Job drawing, mm, ordinate dimensions from the low corner. One solid piece. Round coordinates to 2 decimals unless told otherwise and drop trailing zeros. Write each loop counter-clockwise with the first axis right and the second up, starting at its lowest first coordinate (ties: lowest second). Pieces come first, ordered by that corner, then holes. Notation, with made-up numbers: (21, 63) -> (26, 63) arc R11 cw to (26, 83) -> close; hole circle Ø11 at (29, 5.5). An arc over 180 degrees is marked (long way). Use CSV: the item, a comma, the result in double quotes. Start each with the question number.
(1) Drop flat-ended pins along their axis: pin 1 (1.5 mm diameter, centred on y = 14.5, z = 10, fed in from +X); pin 2 (4 mm diameter, centred on x = 6.5, z = 11.5, fed in from +Y). Give the stop position or say it passes through.
(2) Saw through at A-A (z = 8.5). Give the cut face in (x, y).
(3) Saw through at C-C (y = 16.5). Give the cut face in (x, z), plus the area to 3 significant figures.
(4) Two-plate mould, pull along Z, no slides. Class the marked faces 1, 2 and 3: released by +Z, released by -Z, zero draft, split by the parting line, or undercut.
(5) Probe line 1 (Z direction, x = 2.25, y = 16.5); line 2 (Y direction, x = 0.6, z = 8.5). List the from-to ranges inside material, lowest first. Write a range as [from, to].
(6) Saw through at B-B (x = 11). Give the cut face in (y, z), plus the area to 3 significant figures.
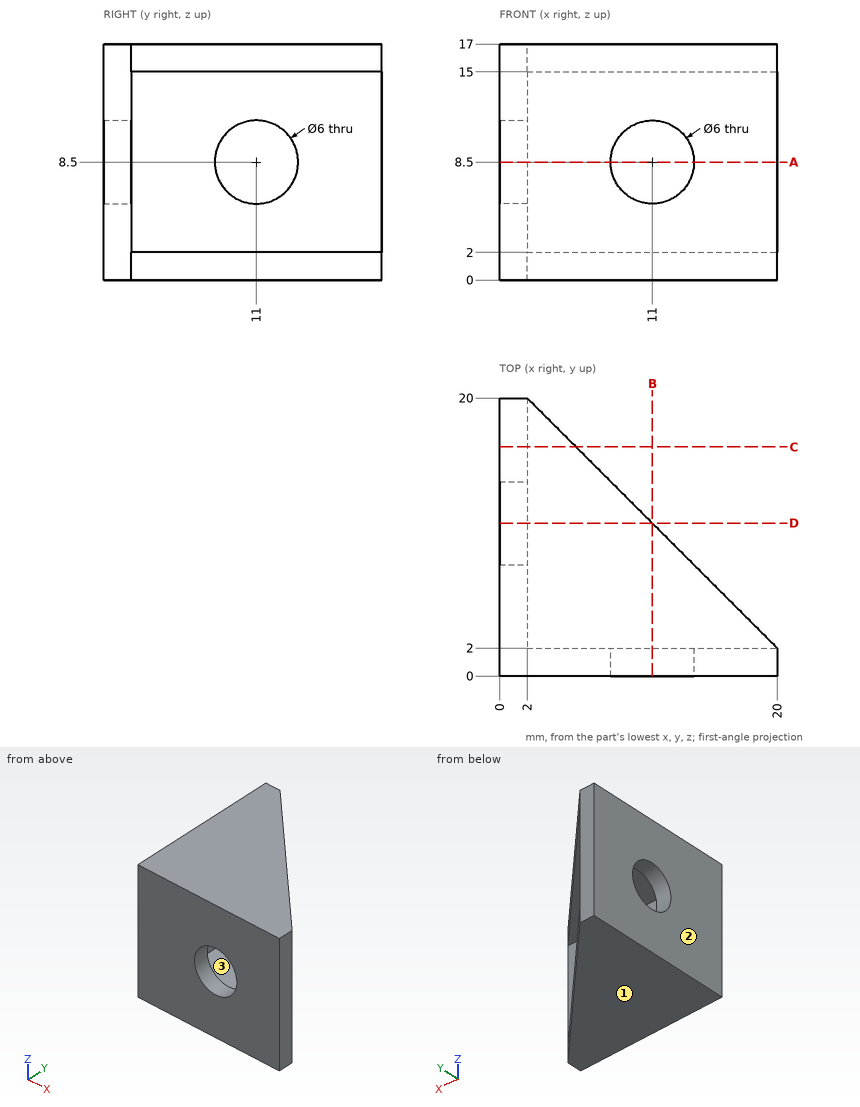
Answers:
1,pin 1,"stops at x = 2"
1,pin 2,"stops at y = 2"
2,outline,"(0, 0) -> (8, 0) -> (8, 2) -> (2, 2) -> (2, 8) -> (0, 8) -> close; (0, 14) -> (2, 14) -> (2, 20) -> (0, 20) -> close; (14, 0) -> (20, 0) -> (20, 2) -> (14, 2) -> close"
3,outline,"(0, 0) -> (5.5, 0) -> (5.5, 2) -> (2, 2) -> (2, 15) -> (5.5, 15) -> (5.5, 17) -> (0, 17) -> close"
3,area,"48.0 mm²"
4,face 1,"released by -Z"
4,face 2,"zero draft"
4,face 3,"undercut"
5,line 1,"z = [0, 2], [15, 17]"
5,line 2,"y = [0, 8], [14, 20]"
6,outline,"(0, 0) -> (11, 0) -> (11, 2) -> (2, 2) -> (2, 5.5) -> (0, 5.5) -> close; (0, 11.5) -> (2, 11.5) -> (2, 15) -> (11, 15) -> (11, 17) -> (0, 17) -> close"
6,area,"58.0 mm²"
